Design review of the part shown in the three views and the two pictorial views. Dimensions are in mm from the part's minimum x, y and z. A direction names the side the tool comes from. Coordinates: 2 decimals unless noted, no trailing zeros. Loops run counter-clockwise (first coordinate to the right, second up) from the corner with the lowest first, then second, coordinate; pieces in that order, holes last. Notation, with made-up numbers: (-13, 27) -> (20, 27) arc R14 cw to (20, 39) -> close; hole circle Ø2 at (14.25, 39). An arc over 180 degrees is marked (long way). Use a Markdown table: item, result. Add a question column.
Q1. For probe 1 along X at (y, z) = (12, 6); probe 2 along Z at (x, y) = (13.97, 10.75) (3 decimals); probe 3 along Z at (x, y) = (13.97, 24), list the stretches that pass through material, from the lowest coordinate up.
Q2. Take a section at D-D on x = 67.5. Write out the cut boundary in (y, z), plus the area to 3 significant figures.
Q3. Take a section at C-C on y = 15.25. Write out the cut boundary in (x, z) (3 decimals).
Q4. Clearance check with flat-ended pins moving along their axes: pin 1 Ø1.9 at (x, z) = (13.5, 5) entering from +Y; pin 2 Ø5 at (y, z) = (4.5, 7.5) entering from -X; pin 3 Ø7.5 at (y, z) = (14, 7.5) entering from -X. State where each tip first meets the part, or that it passes through.
Q5. For the marked faces 4 and 5, list the 3-axis set-ups (+Z, -Z, +X, -X, +Y, -Y) from which the entire face can be reached by the end or side of a thin tool; tool diameter is ignored.
Q6. Draft analysis for pull direction Y (two halves, no side actions). For the marked faces 1, 2 and 3, state which applies: pulls with the +Y half, pulls with the -Y half, needs draft (parallel to the pull), parting line crosses it, or undercut.
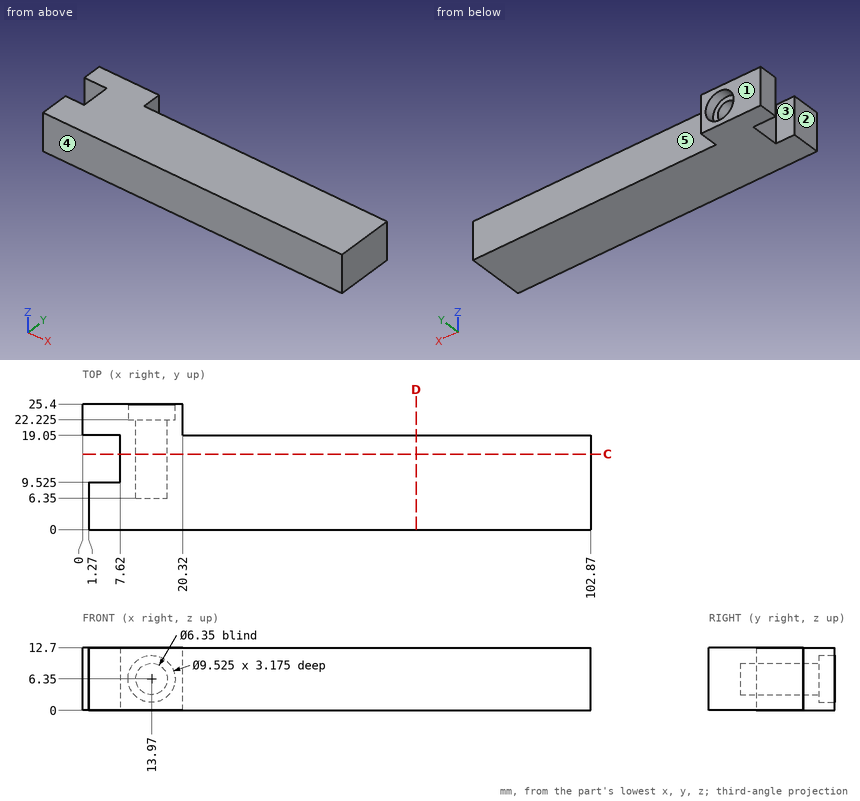
Answer list:
| question | item | result |
|---|---|---|
| 1 | probe 1 | 7.62 to 10.81, 17.13 to 102.87 |
| 1 | probe 2 | 0 to 3.175, 9.525 to 12.7 |
| 1 | probe 3 | 0 to 1.59, 11.11 to 12.7 |
| 2 | outline | (0, 0) -> (19.05, 0) -> (19.05, 12.7) -> (0, 12.7) -> close |
| 2 | area | 242 mm² |
| 3 | outline | (7.62, 0) -> (102.87, 0) -> (102.87, 12.7) -> (7.62, 12.7) -> close; hole circle Ø6.35 at (13.97, 6.35) |
| 4 | pin 1 | y = 6.35 |
| 4 | pin 2 | x = 1.27 |
| 4 | pin 3 | x = 7.62 |
| 5 | face 4 | +Z, -Z, +X, -X, -Y |
| 5 | face 5 | +Z, -Z, +X, +Y |
| 6 | face 1 | pulls with the +Y half |
| 6 | face 2 | needs draft |
| 6 | face 3 | undercut |
